```python
from build123d import *

# Parameters (mm, degrees)
F0_W      = 10
F0_H      = 10
F0_R      = 2.18110555
F1_DEPTH  = 50
F2_R      = 2.18110555
F2_R_2    = 1.75
F3_DEPTH  = 45
F4_W      = 35
F4_H      = 10
F5_DEPTH  = 5
F7_W      = 3
F7_H      = 10
F8_DEPTH  = 15
F9_R      = 1.75
F10_DEPTH = 39.501


# Not quite as in the source:
# - a feature names something its author has since deleted; it is built from what else it names


with BuildPart() as f1:
    # F0 (on Front) → F1 (new body)
    with BuildSketch(Plane.XZ):
        with Locations((-24.531819516, -5.3058740483)):
            Rectangle(F0_W, F0_H)
        with Locations((-24.531819516, -5.3058740483)):
            Circle(F0_R, mode=Mode.SUBTRACT)
    extrude(amount=-F1_DEPTH)

    # F2 (on face) → F3 (cut)
    with BuildSketch(Plane.XZ):
        Polygon((-22.1752951329, -7.844927579), (-21.1546724653, -4.5345908332), (-23.5111968485, -1.9955373025), (-26.8883438992, -2.7668205176), (-27.9089665667, -6.0771572634), (-25.5524421836, -8.6162107941), align=None)
        with Locations((-24.531819516, -5.3058740483)):
            Circle(F2_R, mode=Mode.SUBTRACT)
        Polygon((36.9860127402, -8.419743866), (38.9237869783, -5.5483276646), (37.4059547221, -2.4344578468), (33.9503482277, -2.1920042306), (32.0125739896, -5.063420432), (33.5304062458, -8.1772902498), align=None)
        with Locations((35.468180484, -5.3058740483)):
            Circle(F2_R_2, mode=Mode.SUBTRACT)
    extrude(amount=-F3_DEPTH, mode=Mode.SUBTRACT)

    # F4 (on face) → F5 (join)
    with BuildSketch(Plane.XZ):
        with Locations((-12.031819516, -5.3058740483)):
            Rectangle(F4_W, F4_H)
        Polygon((-22.1752951329, -7.844927579), (-25.5524421836, -8.6162107941), (-27.9089665667, -6.0771572634), (-26.8883438992, -2.7668205176), (-23.5111968485, -1.9955373025), (-21.1546724653, -4.5345908332), align=None, mode=Mode.SUBTRACT)
    extrude(amount=F5_DEPTH)

    # F6: F1 across face


with BuildPart() as f1_1:
    add(f1.part)
    add(f1.part.mirror(Plane(origin=(5.468180484, -2.5, -5.3058740483), x_dir=(0, 1, 0), z_dir=(1, 0, 0))))

    # F7 (on face) → F8 (join)
    with BuildSketch(Plane.XZ.offset(5)):
        with Locations((8.468180484, -5.3058740483)):
            Rectangle(F7_W, F7_H)
        with Locations((2.468180484, -5.3058740483)):
            Rectangle(F7_W, F7_H)
    extrude(amount=F8_DEPTH)

    # F9 (on face) → F10 (cut, through all)
    with BuildSketch(Plane.YZ.offset(9.968180484)):
        with BuildLine():
            ThreePointArc((-20, -5.3058740483), (-18.5355339059, -1.7703401424), (-15, -0.3058740483))
            Line((-15, -0.3058740483), (-20, -0.3058740483))
            Line((-20, -0.3058740483), (-20, -5.3058740483))
        make_face()
        with Locations((-15, -5.3058740483)):
            Circle(F9_R)
        with BuildLine():
            ThreePointArc((-15, -10.3058740483), (-18.5355339059, -8.8414079542), (-20, -5.3058740483))
            Line((-20, -5.3058740483), (-20, -10.3058740483))
            Line((-20, -10.3058740483), (-15, -10.3058740483))
        make_face()
    extrude(amount=-F10_DEPTH, mode=Mode.SUBTRACT)


solid = f1_1.part
```
Can you work these out from the model? Positions are in its coordinate system, mm. A direction names the side the tool comes from. Coordinates: 2 decimals unless noted, no trailing zeros. Order: outer loops, then holes, each group sorted by start corner. A loop starts at its lowest first (then second) coordinate and runs counter-clockwise, first axis right, second up. Notation, with made-up numbers: (8.25, 76) - (17.25, 76) arc R10 cw to (17.25, 85) - close; hole circle Ø3 at (48, -3). An arc over 180 degrees is marked (long way). Answer in a Markdown table with one row per item.
1. Suppose I cut it at B-B (x = -1.5). Please give me the cut outline in (y, z).
Reply:
| item | result |
|---|---|
| outline | (-5, -10.31) - (0, -10.31) - (0, -0.31) - (-5, -0.31) - close |
2. If I drill on line 1 along X through (y, z) = (21.5, -7.75); line 2 along Z through (x, y) = (8.05, -15); line 3 along X through (y, z) = (15, -3.5), over which ranges is the centre line in solid material (lowest first)?
Reply:
| item | result |
|---|---|
| line 1 | x = -29.53 to -26.36, -22.15 to -19.53, 30.47 to 33.08, 37.29 to 40.47 |
| line 2 | z = -10.31 to -7.06, -3.56 to -0.31 |
| line 3 | x = -29.53 to -27.11, -22.11 to -19.53, 30.47 to 33.05, 38.05 to 40.47 |
3. For faces 4 (the flat face through (-19.532, 25, -5)), 5 (the flat face through (-22, 45, -5)), 6 (the flat face through (0.968, -12, -5)), which set-ups out of +Z, -Z, +X, -X, +Y, -Y let a thin tool reach every point of the face, with its end or its side?
Reply:
| item | result |
|---|---|
| face 4 | +Z, -Z, +Y |
| face 5 | -Y |
| face 6 | +Z, -Z, -X, -Y |
4. For pin 1 (2 mm diameter, centred on x = 10, z = -2, fed in from -Y); pin 2 (3 mm diameter, centred on x = 23.5, z = -5.5, fed in from -Y); pin 3 (1 mm diameter, centred on x = -3, y = -6.5, fed in from -Z); pin 4 (3.5 mm diameter, centred on x = 6, z = -4, fed in from -Y), each with a flat end and sliding along its axis, tell me the tip position at first contact or that it passes through.
Reply:
| item | result |
|---|---|
| pin 1 | stops at y = -19.44 |
| pin 2 | stops at y = -5 |
| pin 3 | passes through |
| pin 4 | stops at y = -20 |
5. If we mould it in two halves opening along X, with no side actions, what happens to faces 1 (the flat face through (38.342, 20.35, -4.445)), 2 (the flat face through (-14, -5, -5)), 3 (the flat face through (-29.532, 23, -5))? For each: pulls with the +X half, pulls with the -X half, needs draft (parallel to the pull), parting line crosses it, or undercut.
Reply:
| item | result |
|---|---|
| face 1 | undercut |
| face 2 | needs draft |
| face 3 | pulls with the -X half |
6. Suppose I cut it at A-A (y = 46). Please give me the cut outline in (x, z), and give its area (3 significant figures).
Reply:
| item | result |
|---|---|
| outline | (-29.53, -10.31) - (-19.53, -10.31) - (-19.53, -0.31) - (-29.53, -0.31) - close; (30.47, -10.31) - (40.47, -10.31) - (40.47, -0.31) - (30.47, -0.31) - close; hole circle Ø4.36 at (-24.53, -5.31); hole circle Ø4.36 at (35.47, -5.31) |
| area | 170 mm^2 |
